Design review of the part built by this model. Coordinates are the model's own, in mm. Face numbers are marked on the shaded views. A direction names the side the tool comes from. Coordinates: 2 decimals unless noted, no trailing zeros. Write each loop counter-clockwise with the first axis right and the second up, starting at its lowest first coordinate (ties: lowest second). Pieces come first, ordered by that corner, then holes.
Q1. Machinability: for the marked faces 1 and 2, which of the approach directions +Z, -Z, +X, -X, +Y, -Y give a long, thin tool a straight path to every point of the face, cutting with its end or side? Answer none if there is none.
Q2. The part is to be moulded in two halves that separate along X. For the marked faces 3, 4 and 5, say which applies: +X half, -X half, draft (parallel to the pull), parting line (faces both ways), or undercut.
Q3. To check wall thickness, follow probe 1 along X at (y, z) = (2.75, -0.1); probe 2 along Y at (x, z) = (-16.5, -0.3); probe 3 along Y at (x, z) = (-7, -0.45). State the ranges of each line that lie inside material, in increasing order.
Q4. Add section C-C, the plane z = -0.3. Give the number of separate pieces and of enclosed holes in the cut face, plus the area to 3 significant figures.
Q5. Add section B-B, the plane x = -18.25. Give the boundary of the cut face in (y, z).
Q6. Add section A-A, the plane y = -2. Give the boundary of the cut face in (x, z).
Q7. Clearance check with flat-ended pins moving along their axes: pin 1 Ø0.6 at (x, z) = (-4, -0.5) entering from +Y; pin 2 Ø10 at (x, y) = (-9.5, -6) entering from -Z; pin 3 Ø0.6 at (x, z) = (-4.5, -0.5) entering from -Y; pin 4 Ø4.5 at (x, y) = (-13.5, 3.5) entering from -Z. State where each tip first meets the part, or that it passes through.
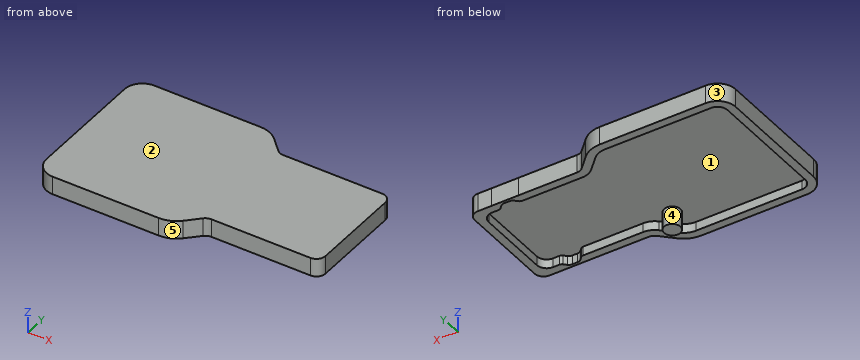
from build123d import *

# Parameters (mm, degrees)
EXTRUDE_1_DEPTH = 1
EXTRUDE_START   = 1
EXTRUDE_2_DEPTH = 1
EXTRUDE_3_DEPTH = 2
FILLET_1_R      = 1


with BuildPart() as part:
    # 草图1 → 凸台-拉伸1 (new body)
    with BuildSketch(Plane.XY):
        with BuildLine():
            ThreePointArc((-11.921595121, -5.987310135), (-12.309141559, -6.064397915), (-12.637687565, -6.283925339))
            Line((-12.637687565, -6.283925339), (-13.9661153, -7.612353074))
            ThreePointArc((-13.9661153, -7.612353074), (-14.935267633, -8.259919962), (-16.078460757, -8.487315215))
            Line((-16.078460757, -8.487315215), (-27.75005588, -8.487315215))
            ThreePointArc((-27.75005588, -8.487315215), (-29.155290964, -7.905247784), (-29.737358395, -6.5000127))
            Line((-29.737358395, -6.5000127), (-29.737358395, 6.5000127))
            ThreePointArc((-29.737358395, 6.5000127), (-29.155290964, 7.905247784), (-27.75005588, 8.487315215))
            Line((-27.75005588, 8.487315215), (-16.078460755, 8.487315215))
            ThreePointArc((-16.078460755, 8.487315215), (-14.935267633, 8.259919962), (-13.966115301, 7.612353076))
            Line((-13.966115301, 7.612353076), (-12.637687563, 6.283925337))
            ThreePointArc((-12.637687563, 6.283925337), (-12.309141741, 6.06439799), (-11.921595517, 5.987310135))
            Line((-11.921595517, 5.987310135), (-5.508963215, 5.987312659))
            Line((-5.508963215, 5.987312659), (-2.49105204, 5.987310135))
            Line((-2.49105204, 5.987310135), (-2.00000508, 5.987310135))
            Line((-2.00000508, 5.987310135), (-0.012702565, 5.987310135))
            Line((-0.012702565, 5.987310135), (-0.012702565, 4.00000762))
            Line((-0.012702565, 4.00000762), (-0.012702565, -4.00000762))
            Line((-0.012702565, -4.00000762), (-0.012702565, -5.987310135))
            Line((-0.012702565, -5.987310135), (-2.00000508, -5.987310135))
            Line((-2.00000508, -5.987310135), (-2.49105458, -5.987310135))
            Line((-2.49105458, -5.987310135), (-5.5089632, -5.987310135))
            Line((-5.5089632, -5.987310135), (-11.921595121, -5.987310135))
        make_face()
    extrude(amount=EXTRUDE_1_DEPTH)

    # 草图2 → 凸台-拉伸2 (add)
    with BuildSketch(Plane(origin=(0, 0, 0), x_dir=(-1, 0, 0), z_dir=(0, 0, -1)).offset(EXTRUDE_START)):
        with BuildLine():
            Line((0.012702565, -5.987310135), (11.921595121, -5.987310135))
            ThreePointArc((11.921595121, -5.987310135), (12.309141559, -6.064397915), (12.637687565, -6.283925339))
            Line((12.637687565, -6.283925339), (13.9661153, -7.612353074))
            ThreePointArc((13.9661153, -7.612353074), (14.935267633, -8.259919962), (16.078460757, -8.487315215))
            Line((16.078460757, -8.487315215), (27.75005588, -8.487315215))
            ThreePointArc((27.75005588, -8.487315215), (29.155290964, -7.905247784), (29.737358395, -6.5000127))
            Line((29.737358395, -6.5000127), (29.737358395, 6.5000127))
            ThreePointArc((29.737358395, 6.5000127), (29.155290964, 7.905247784), (27.75005588, 8.487315215))
            Line((27.75005588, 8.487315215), (16.078460755, 8.487315215))
            ThreePointArc((16.078460755, 8.487315215), (14.935267633, 8.259919962), (13.966115301, 7.612353076))
            Line((13.966115301, 7.612353076), (12.637687563, 6.283925337))
            ThreePointArc((12.637687563, 6.283925337), (12.309141741, 6.06439799), (11.921595517, 5.987310135))
            Line((11.921595517, 5.987310135), (5.508963215, 5.987312659))
            Line((5.508963215, 5.987312659), (2.49105204, 5.987310135))
            Line((2.49105204, 5.987310135), (0.012702565, 5.987310135))
            Line((0.012702565, 5.987310135), (0.012702565, -5.987310135))
        make_face()
        with BuildLine():
            Line((0.912702565, -4.00000762), (0.912702565, 4.00000762))
            ThreePointArc((0.912702565, 4.00000762), (1.231166099, 4.768846601), (2.00000508, 5.087310135))
            Line((2.00000508, 5.087310135), (2.692900097, 5.087310135))
            ThreePointArc((2.692900097, 5.087310135), (2.850834155, 5.118726257), (2.984723794, 5.208189682))
            Line((2.984723794, 5.208189682), (3.291830699, 5.515296587))
            ThreePointArc((3.291830699, 5.515296587), (3.482364562, 5.642607176), (3.707114551, 5.687312675))
            Line((3.707114551, 5.687312675), (4.292903203, 5.687312675))
            ThreePointArc((4.292903203, 5.687312675), (4.517653218, 5.642607176), (4.708187099, 5.515296569))
            Line((4.708187099, 5.515296569), (5.015294015, 5.208189653))
            ThreePointArc((5.015294015, 5.208189653), (5.149076381, 5.118771977), (5.306884994, 5.087312733))
            Line((5.306884994, 5.087312733), (11.921595123, 5.087310135))
            ThreePointArc((11.921595123, 5.087310135), (12.653556649, 5.232906336), (13.274083668, 5.647529236))
            Line((13.274083668, 5.647529236), (14.602511404, 6.975956972))
            ThreePointArc((14.602511404, 6.975956972), (15.279682723, 7.428428383), (16.078460757, 7.587315215))
            Line((16.078460757, 7.587315215), (27.75005588, 7.587315215))
            ThreePointArc((27.75005588, 7.587315215), (28.518894861, 7.268851681), (28.837358395, 6.5000127))
            Line((28.837358395, 6.5000127), (28.837358395, -6.5000127))
            ThreePointArc((28.837358395, -6.5000127), (28.518894861, -7.268851681), (27.75005588, -7.587315215))
            Line((27.75005588, -7.587315215), (16.078460757, -7.587315215))
            ThreePointArc((16.078460757, -7.587315215), (15.279682723, -7.428428383), (14.602511404, -6.975956973))
            Line((14.602511404, -6.975956973), (13.274083667, -5.647529236))
            ThreePointArc((13.274083667, -5.647529236), (12.653556649, -5.232906336), (11.921595123, -5.087310135))
            Line((11.921595123, -5.087310135), (5.307117071, -5.087310135))
            ThreePointArc((5.307117071, -5.087310135), (5.149183592, -5.118725011), (5.015294034, -5.208187095))
            Line((5.015294034, -5.208187095), (4.708187081, -5.515294047))
            ThreePointArc((4.708187081, -5.515294047), (4.517653218, -5.642604636), (4.292903229, -5.687310135))
            Line((4.292903229, -5.687310135), (3.707114577, -5.687310135))
            ThreePointArc((3.707114577, -5.687310135), (3.482364562, -5.642604636), (3.291830681, -5.515294029))
            Line((3.291830681, -5.515294029), (2.984723765, -5.208187113))
            ThreePointArc((2.984723765, -5.208187113), (2.850834188, -5.118725011), (2.692900682, -5.087310135))
            Line((2.692900682, -5.087310135), (2.00000508, -5.087310135))
            ThreePointArc((2.00000508, -5.087310135), (1.231166099, -4.768846601), (0.912702565, -4.00000762))
        make_face(mode=Mode.SUBTRACT)
    extrude(amount=-EXTRUDE_2_DEPTH)

    # 草图2<4> → 凸台-拉伸3 (add)
    with BuildSketch(Plane(origin=(0, 0, 0), x_dir=(-1, 0, 0), z_dir=(0, 0, -1))):
        with BuildLine():
            ThreePointArc((14.197426975, -5.123210566), (15.097429515, -6.023213106), (15.997432055, -5.123210566))
            ThreePointArc((15.997432055, -5.123210566), (15.097429515, -4.223208026), (14.197426975, -5.123210566))
        make_face()
    extrude(amount=EXTRUDE_3_DEPTH)

    # 圆角1
    fillet_1_edges = [part.edges().sort_by_distance(p)[0] for p in [
        (-0.012702565, 5.987310135, 0),
        (-0.012702565, -5.987310135, 0),
    ]]
    fillet(fillet_1_edges, radius=FILLET_1_R)


solid = part.part
Here are the results:
1. face 1: -Z
1. face 2: +Z, +X, -X, +Y, -Y
2. face 3: -X half
2. face 4: undercut
2. face 5: +X half
3. probe 1: x = -29.74 to -28.84, -0.91 to -0.01
3. probe 2: y = -8.49 to -7.59, 7.59 to 8.49
3. probe 3: y = -5.99 to -5.09, 5.09 to 5.99
4. separate pieces: 2
4. enclosed holes: 1
4. area: 77.3 mm2
5. outline: (-8.49, -1) - (-7.59, -1) - (-7.59, 0) - (7.59, 0) - (7.59, -1) - (8.49, -1) - (8.49, 1) - (-8.49, 1) - close
6. outline: (-29.74, -1) - (-28.84, -1) - (-28.84, 0) - (-0.91, 0) - (-0.91, -1) - (-0.01, -1) - (-0.01, 1) - (-29.74, 1) - close
7. pin 1: stops at y = 5.99
7. pin 2: stops at z = -2
7. pin 3: stops at y = -5.99
7. pin 4: stops at z = -1
